from build123d import *

# Parameters (mm, degrees)
SKETCH1_W                      = 88.9
SKETCH1_H                      = 88.9
BOSS_EXTRUDE1_DEPTH            = 21.082
CUT_EXTRUDE1_DEPTH             = 0.5
SKETCH3_W                      = 54.9
SKETCH3_H                      = 54.9
CUT_EXTRUDE2_DEPTH             = 3
FILLET1_R                      = 6.35
CBORE_FOR_M6_SHCS1_D           = 6.6
CBORE_FOR_M6_SHCS1_CBORE_D     = 11
CBORE_FOR_M6_SHCS1_CBORE_DEPTH = 14.7376
M5X0_8_TAPPED_HOLE1_D          = 4.2


with BuildPart() as part:
    # Sketch1 → Boss-Extrude1 (new body)
    with BuildSketch(Plane(origin=(0, 0, 0), x_dir=(1, 0, 0), z_dir=(0, 1, 0))):
        Rectangle(SKETCH1_W, SKETCH1_H)
    extrude(amount=BOSS_EXTRUDE1_DEPTH)

    # Sketch2 → Cut-Extrude1 (cut)
    with BuildSketch(Plane(origin=(0, 21.082, 0), x_dir=(1, 0, 0), z_dir=(0, 1, 0))):
        with BuildLine():
            Line((28.134397615, -32.45), (-28.134397615, -32.45))
            ThreePointArc((-28.134397615, -32.45), (-33.157106781, -33.157106781), (-32.45, -28.134397615))
            Line((-32.45, -28.134397615), (-32.45, 28.134397615))
            ThreePointArc((-32.45, 28.134397615), (-33.157106781, 33.157106781), (-28.134397615, 32.45))
            Line((-28.134397615, 32.45), (28.134397615, 32.45))
            ThreePointArc((28.134397615, 32.45), (33.157106781, 33.157106781), (32.45, 28.134397615))
            Line((32.45, 28.134397615), (32.45, -28.134397615))
            ThreePointArc((32.45, -28.134397615), (33.157106781, -33.157106781), (28.134397615, -32.45))
        make_face()
    extrude(amount=-CUT_EXTRUDE1_DEPTH, mode=Mode.SUBTRACT)

    # Sketch3 → Cut-Extrude2 (cut)
    with BuildSketch(Plane(origin=(0, 20.582, 0), x_dir=(1, 0, 0), z_dir=(0, 1, 0))):
        Rectangle(SKETCH3_W, SKETCH3_H)
    extrude(amount=-CUT_EXTRUDE2_DEPTH, mode=Mode.SUBTRACT)

    # Fillet1
    fillet1_edges = [part.edges().sort_by_distance(p)[0] for p in [
        (27.45, 19.082, 27.45),
        (-27.45, 19.082, 27.45),
        (-27.45, 19.082, -27.45),
        (27.45, 19.082, -27.45),
    ]]
    fillet(fillet1_edges, radius=FILLET1_R)

    # CBORE for M6 SHCS1 (through all)
    with Locations(Plane(origin=(0, 21.082, 0), x_dir=(1, 0, 0), z_dir=(0, 1, 0))):
        with Locations((-25, 25), (25, 25), (25, -25), (-25, -25)):
            CounterBoreHole(CBORE_FOR_M6_SHCS1_D / 2, CBORE_FOR_M6_SHCS1_CBORE_D / 2, CBORE_FOR_M6_SHCS1_CBORE_DEPTH)

    # M5x0.8 Tapped Hole1 (through all)
    with Locations(Plane(origin=(0, 21.082, 0), x_dir=(1, 0, 0), z_dir=(0, 1, 0))):
        with Locations((-38.45, 22.523488527), (-38.45, 0), (-38.45, -22.523488527), (-22.523488527, -38.45), (0, -38.45), (22.523488527, -38.45), (38.45, -22.523488527), (38.45, 0), (38.45, 22.523488527), (22.523488527, 38.45), (0, 38.45), (-22.523488527, 38.45)):
            Hole(M5X0_8_TAPPED_HOLE1_D / 2)


solid = part.part
Source: CAD feature listing. Evaluate the final solid. Frame: model axes, mm. A direction names the side the tool comes from. Give positions to 0.01 mm unless a question says otherwise; leave off trailing zeros. Write each loop counter-clockwise with the first axis right and the second up, starting at its lowest first coordinate (ties: lowest second). Pieces come first, ordered by that corner, then holes. Notation, with made-up numbers: (84.5, 38.5) - (139.5, 38.5) arc R25 cw to (139.5, 52.5) - close; hole circle Ø10 at (54.5, 42). An arc over 180 degrees is marked (long way). Write item = value, one per line. Start each with the question number.
Q1. Material intervals for probe 1 along X at (y, z) = (4, 25); probe 2 along Z at (x, y) = (-38.45, 14.75), sorted ascending.
Q2. Cut plane B-B, the plane x = 38.45. Return loops of the section in (y, z).
Q3. Draft query along Z for faces 1 (the cylindrical face through (33.215, 20.836, 33.098)), 2 (the flat face through (-1, 10, -44.45)), 3 (the flat face through (-1, 0, -1)). Return one class per face: +Z half, -Z half, draft (parallel to the pull), parting line (faces both ways), or undercut.
Q4. Cut plane D-D, the plane z = 11.5. Return loops of the section in (x, y), then the cut area to 3 significant figures.
Q5. Cut plane A-A, the plane z = -38.45. Return loops of the section in (x, y), then the cut area to 3 significant figures.
Q6. Pin query (flat end, axial travel): pin 1 Ø6.5 at (x, z) = (38.45, 0) entering from -Y; pin 2 Ø3 at (x, z) = (23, 21) entering from +Y; pin 3 Ø4 at (x, z) = (30.91, -30.91) entering from +Y; pin 4 Ø8.5 at (x, z) = (25, -25) entering from +Y. Return the tip coordinate at first contact, or that it passes through.
Q7. Reachability of faces 4 (the cylindrical face through (-28.05, 3.13, 26.26)), 5 (the flat face through (-27.45, 19, 0)) from +Z, -Z, +X, -X, +Y, -Y: full face, straight path, thin tool, end or side. Return the list, or none.
Q8. Cut plane C-C, the plane y = 18.75. Give the number of separate pieces and of enclosed holes in the cut face, then the cut area to 3 significant figures.
Computed values:
q1.probe_1 = -44.45 to -28.3, -21.7 to 21.7, 28.3 to 44.45
q1.probe_2 = -44.45 to -24.62, -20.42 to -2.1, 2.1 to 20.42, 24.62 to 44.45
q2.outline = (0, -44.45) - (21.08, -44.45) - (21.08, -24.62) - (0, -24.62) - close; (0, -20.42) - (21.08, -20.42) - (21.08, -2.1) - (0, -2.1) - close; (0, 2.1) - (21.08, 2.1) - (21.08, 20.42) - (0, 20.42) - close; (0, 24.62) - (21.08, 24.62) - (21.08, 44.45) - (0, 44.45) - close
q3.face_1 = undercut
q3.face_2 = -Z half
q3.face_3 = draft
q4.outline = (-44.45, 0) - (44.45, 0) - (44.45, 21.08) - (32.45, 21.08) - (32.45, 20.58) - (27.45, 20.58) - (27.45, 17.58) - (-27.45, 17.58) - (-27.45, 20.58) - (-32.45, 20.58) - (-32.45, 21.08) - (-44.45, 21.08) - close
q4.area = 1,680 mm²
q5.outline = (-44.45, 0) - (-24.62, 0) - (-24.62, 21.08) - (-44.45, 21.08) - close; (-20.42, 0) - (-2.1, 0) - (-2.1, 21.08) - (-20.42, 21.08) - close; (2.1, 0) - (20.42, 0) - (20.42, 21.08) - (2.1, 21.08) - close; (24.62, 0) - (44.45, 0) - (44.45, 21.08) - (24.62, 21.08) - close
q5.area = 1,610 mm²
q6.pin_1 = 0
q6.pin_2 = 17.58
q6.pin_3 = 20.58
q6.pin_4 = 6.34
q7.face_4 = +Y, -Y
q7.face_5 = +Y
q8.separate_pieces = 1
q8.enclosed_holes = 13
q8.area = 4,570 mm²
